```python
from build123d import *

# Parameters (mm, degrees)
SKETCH1_R               = 4.765
BOSS_EXTRUDE1_DEPTH     = 19.05
CHAMFER1_SIZE           = 0.76
CUT_EXTRUDE1_DEPTH      = 21.206755059
CUT_EXTRUDE1_DEPTH_BACK = 21.206755059
SKETCH2_R               = 3.43


with BuildPart() as part:
    # Sketch1 → Boss-Extrude1 (new body)
    with BuildSketch(Plane(origin=(0, 0, 0), x_dir=(0, 0, -1), z_dir=(1, 0, 0))):
        with Locations(Location((0, 0, 0), (0, 0, 180))):
            Circle(SKETCH1_R)
    extrude(amount=BOSS_EXTRUDE1_DEPTH)

    # Chamfer1
    chamfer1_edges = [part.edges().sort_by_distance(p)[0] for p in [
        (0, 0, -4.765),
        (19.05, 0, -4.765),
    ]]
    chamfer(chamfer1_edges, length=CHAMFER1_SIZE)

    # Sketch2 → Cut-Extrude1 (cut, two sides: drawn at the far end of the back side and taken through both)
    with BuildSketch(Plane(origin=(0, 0, 0), x_dir=(1, 0, 0), z_dir=(0, 1, 0)).offset(-CUT_EXTRUDE1_DEPTH_BACK)):
        with Locations(Location((9.525, 0, 0), (0, 0, 270))):
            Circle(SKETCH2_R)
    extrude(amount=CUT_EXTRUDE1_DEPTH + CUT_EXTRUDE1_DEPTH_BACK, mode=Mode.SUBTRACT)


solid = part.part
```
Build history of the part. All positions in model axes, mm. Give positions to 0.01 mm unless a question says otherwise; leave off trailing zeros. Loops run counter-clockwise (first coordinate to the right, second up) from the corner with the lowest first, then second, coordinate; pieces in that order, holes last.
1) Drop flat-ended pins along their axis: P1, Ø4, axis at x = 12.5, y = -3.5, coming from the +Z side; P2, Ø3, axis at x = 17, z = -3.5, coming from the +Y side; P3, Ø2, axis at x = 9, y = 2.5, coming from the -Z side. Give the stop position or say it passes through.
Values follow:
P1: stops at z = 4.52
P2: stops at y = 4.32
P3: stops at z = -4.52
2) Band-saw the part on B-B on y = 0. List the corners of the cut face in (x, z) (3 decimals), then the cut area to 3 significant figures.
Values follow:
outline: (0, -4.005) - (0.76, -4.765) - (18.29, -4.765) - (19.05, -4.005) - (19.05, 4.005) - (18.29, 4.765) - (0.76, 4.765) - (0, 4.005) - close; hole circle Ø6.86 at (9.525, 0)
area: 143 mm2
3) Band-saw the part on A-A on z = 0. List the corners of the cut face in (x, y) (3 decimals).
Values follow:
outline: (0, -4.005) - (0.76, -4.765) - (6.095, -4.765) - (6.095, 4.765) - (0.76, 4.765) - (0, 4.005) - close; (12.955, -4.765) - (18.29, -4.765) - (19.05, -4.005) - (19.05, 4.005) - (18.29, 4.765) - (12.955, 4.765) - close
4) Probe line 1 along X through (y, z) = (1.75, 0) (3 decimals); line 2 along Z through (x, y) = (6.5, 2.5); line 3 along Z through (x, y) = (7.25, 0.25). List the from-to ranges inside material, lowest first.
Values follow:
line 1: x = 0 to 6.095, 12.955 to 19.05
line 2: z = -4.06 to -1.62, 1.62 to 4.06
line 3: z = -4.76 to -2.57, 2.57 to 4.76
5) Band-saw the part on C-C on x = 15.5. List the corners of the cut face in (y, z) (3 decimals), then the cut area to 3 significant figures.
Values follow:
outline: circle Ø9.53 at (0, 0)
area: 71.3 mm2
